```python
from build123d import *

# Parameters (mm, degrees)
SKETCH_3_R               = 5.5
EXTRUDE_1_DEPTH          = 10
SKETCH_4_R               = 1.5
CUT_EXTRUDE_1_DEPTH      = 45.55333882
CUT_EXTRUDE_2_DEPTH      = 45.55333882
CUT_EXTRUDE_2_DEPTH_BACK = 45.55333882
SKETCH_5_R               = 1.5


with BuildPart() as part:
    # Эскиз3 → Бобышка-Вытянуть1 (new body)
    with BuildSketch(Plane.XY):
        with BuildLine():
            Line((-17, 0), (-17, -17))
            Line((-17, -17), (-27, -17))
            Line((-27, -17), (-27, -22))
            Line((-27, -22), (27, -22))
            Line((27, -22), (27, -17))
            Line((27, -17), (17, -17))
            Line((17, -17), (17, 0))
            ThreePointArc((17, 0), (0, 17), (-17, 0))
        make_face()
        Circle(SKETCH_3_R, mode=Mode.SUBTRACT)
    extrude(amount=EXTRUDE_1_DEPTH)

    # Эскиз4 → Вырез-Вытянуть1 (cut, through all)
    with BuildSketch(Plane(origin=(0, -17, 0), x_dir=(1, 0, 0), z_dir=(0, 1, 0))):
        with Locations(Location((22, -5, 0), (0, 0, 270))):
            Circle(SKETCH_4_R)
    extrude(amount=-CUT_EXTRUDE_1_DEPTH, mode=Mode.SUBTRACT)

    # Эскиз5 → Вырез-Вытянуть2 (cut, two sides: drawn at the far end of the back side and taken through both)
    with BuildSketch(Plane(origin=(0, -17, 0), x_dir=(1, 0, 0), z_dir=(0, 1, 0)).offset(-CUT_EXTRUDE_2_DEPTH_BACK)):
        with Locations(Location((-22, -5, 0), (0, 0, 270))):
            Circle(SKETCH_5_R)
    extrude(amount=CUT_EXTRUDE_2_DEPTH + CUT_EXTRUDE_2_DEPTH_BACK, mode=Mode.SUBTRACT)


solid = part.part
```
Part model, mm, in its own coordinate system. A direction names the side the tool comes from. Coordinates: 2 decimals unless noted, no trailing zeros. Write each loop counter-clockwise with the first axis right and the second up, starting at its lowest first coordinate (ties: lowest second). Pieces come first, ordered by that corner, then holes.
Item 1: Slice it at C-C (z = 9.25). Write the cut outline in (x, y).
Item 2: Slice it at A-A (z = 5). Write the cut outline in (x, y), and give its area (3 significant figures).
Item 3: Pin check, flat tips, straight feed: pin 1 (6 mm diameter, centred on x = 7, y = -6.5, fed in from -Z); pin 2 (4 mm diameter, centred on x = 22, z = 5, fed in from +Y); pin 3 (3 mm diameter, centred on y = -11.5, z = 4, fed in from -X); pin 4 (1 mm diameter, centred on x = -1.5, z = 6, fed in from +Y). Stop position of each tip, or through.
Item 4: Which spindle directions (+Z, -Z, +X, -X, +Y, -Y) get a long thin tool onto all of the face, cutting with end or side? Do faces 1 (the face through (-17, -8, 5)), 2 (the face through (17, -9, 5)), 3 (the face through (0, -7, 0)). Say none if no direction does.
Item 5: Probe line 1 (X direction, y = -19.75, z = 5); line 2 (Z direction, x = -22, y = -20.6); line 3 (X direction, y = -18.5, z = 4). List the from-to ranges inside material, lowest first.
Item 6: Slice it at B-B (x = 0). Write the cut outline in (y, z), and give its area (3 significant figures).
Item 7: Mould opens along Y. For faces 4 (the face through (-1.19, -5.37, 4.93)), 5 (the face through (23.2, -17, 3.8)), 6 (the face through (23.265, -19.465, 5.806)) say: released by +Y, released by -Y, zero draft, split by the parting line, or undercut.
Item 8: Slice it at D-D (x = 22). Write the cut outline in (y, z), and give its area (3 significant figures).
Results found:
1. outline: (-27, -22) - (27, -22) - (27, -17) - (17, -17) - (17, 0) arc R17 ccw to (-17, 0) - (-17, -17) - (-27, -17) - close; hole circle Ø11 at (0, 0)
2. outline: (-27, -22) - (-23.5, -22) - (-23.5, -17) - (-27, -17) - close; (-20.5, -22) - (20.5, -22) - (20.5, -17) - (17, -17) - (17, 0) arc R17 ccw to (-17, 0) - (-17, -17) - (-20.5, -17) - close; (23.5, -22) - (27, -22) - (27, -17) - (23.5, -17) - close; hole circle Ø11 at (0, 0)
2. area: 1,180 mm2
3. pin 1: stops at z = 0
3. pin 2: stops at y = -17
3. pin 3: stops at x = -17
3. pin 4: stops at y = 16.97
4. face 1: +Z, -Z, -X, +Y
4. face 2: +Z, -Z, +X, +Y
4. face 3: -Z, +X, -X, +Y, -Y
5. line 1: x = -27 to -23.5, -20.5 to 20.5, 23.5 to 27
5. line 2: z = 0 to 3.5, 6.5 to 10
5. line 3: x = -27 to -23.12, -20.88 to 20.88, 23.12 to 27
6. outline: (-22, 0) - (-5.5, 0) - (-5.5, 10) - (-22, 10) - close; (5.5, 0) - (17, 0) - (17, 10) - (5.5, 10) - close
6. area: 280 mm2
7. face 4: undercut
7. face 5: released by +Y
7. face 6: zero draft
8. outline: (-22, 0) - (-17, 0) - (-17, 3.5) - (-22, 3.5) - close; (-22, 6.5) - (-17, 6.5) - (-17, 10) - (-22, 10) - close
8. area: 35.0 mm2
